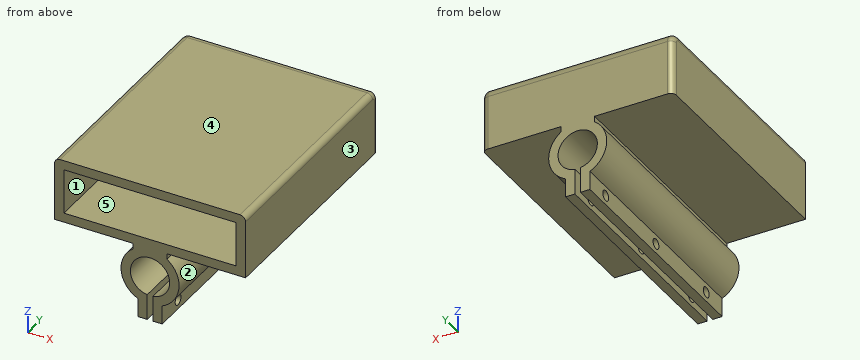
```python
from build123d import *

# Parameters (mm, degrees)
PAD_DEPTH       = 125
SKETCH001_W     = 92
SKETCH001_H     = 24
POCKET_DEPTH    = 120
FILLET_R        = 5
FILLET001_R     = 3
FILLET002_R     = 3
SKETCH002_R     = 2.75
POCKET001_DEPTH = 57.501


with BuildPart() as part:
    # Sketch → Pad (new body)
    with BuildSketch(Plane.XZ):
        with BuildLine():
            ThreePointArc((1.5, -26.011734), (0, -5.119429), (-1.5, -26.011734))
            Line((-1.5, -26.011734), (-1.5, -39.690677))
            Line((-1.5, -39.690677), (-6.5, -39.690677))
            Line((-6.5, -39.690677), (-6.5, -29.690677))
            ThreePointArc((-9, -3), (-15.432451, -17.06492), (-6.5, -29.690677))
            Line((-9, -3), (-9, 0))
            Line((-9, 0), (-51, 0))
            Line((-51, 0), (-51, 34))
            Line((-51, 34), (51, 34))
            Line((51, 0), (51, 34))
            Line((9, 0), (51, 0))
            Line((9, -3), (9, 0))
            ThreePointArc((6.5, -29.690677), (15.432451, -17.06492), (9, -3))
            Line((6.5, -39.690677), (6.5, -29.690677))
            Line((1.5, -39.690677), (6.5, -39.690677))
            Line((1.5, -26.011734), (1.5, -39.690677))
        make_face()
    extrude(amount=PAD_DEPTH)

    # Sketch001 (on Face18 of Pad) → Pocket (cut)
    with BuildSketch(Plane.XZ.offset(125)):
        with Locations((0, 17)):
            Rectangle(SKETCH001_W, SKETCH001_H)
    extrude(amount=-POCKET_DEPTH, mode=Mode.SUBTRACT)

    # Fillet
    fillet_edges = [part.edges().sort_by_distance(p)[0] for p in [
        (0, 0, 34),
    ]]
    fillet(fillet_edges, radius=FILLET_R)

    # Fillet001
    fillet001_edges = [part.edges().sort_by_distance(p)[0] for p in [
        (51, 0, 14.5),
    ]]
    fillet(fillet001_edges, radius=FILLET001_R)

    # Fillet002
    fillet002_edges = [part.edges().sort_by_distance(p)[0] for p in [
        (-51, 0, 14.5),
    ]]
    fillet(fillet002_edges, radius=FILLET002_R)

    # Sketch002 (on Face12 of Fillet002) → Pocket001 (cut, through all)
    with BuildSketch(Plane(origin=(6.5, 0, 0), x_dir=(0, 0, 1), z_dir=(1, 0, 0))):
        with Locations((-34.690677, 110)):
            Circle(SKETCH002_R)
        with Locations((-34.690677, 62.5)):
            Circle(SKETCH002_R)
        with Locations((-34.690677, 15)):
            Circle(SKETCH002_R)
    extrude(amount=-POCKET001_DEPTH, mode=Mode.SUBTRACT)


solid = part.part
```
Check sheet for the modelled part. Datum: model origin and axes. Units: mm. Face numbers are marked on the shaded views. A direction names the side the tool comes from. Round coordinates to 2 decimals unless told otherwise and drop trailing zeros. Order: outer loops, then holes, each group sorted by start corner. A loop starts at its lowest first (then second) coordinate and runs counter-clockwise, first axis right, second up.
1) Section check A-A (y = -110). Give the number of separate pieces and of enclosed holes in the cut face, and give its area (3 significant figures).
2) Tool access check on the marked faces 1 and 2. Record the directions out of +Z, -Z, +X, -X, +Y, -Y that give a thin tool (end or side, any length) a straight path to the whole face; none if there is none.
3) Mould release check, pull along X, two halves, no side actions. Record for the marked faces 3, 4 and 5: +X half, -X half, draft (parallel to the pull), parting line (faces both ways), or undercut.
4) Scan lines: line 1 (X direction, y = -88, z = 19); line 2 (Z direction, x = 30, y = -71); line 3 (X direction, y = -115.5, z = -35.5). Record each from-to range of solid material in increasing order.
5) Section check B-B (y = -25). Record the boundary of the cut face in (x, z), and give its area (3 significant figures).
6) Section check D-D (x = -29.5). Record the boundary of the cut face in (y, z).
7) Section check C-C (z = 13.5). Record the boundary of the cut face in (x, y).
8) Go/stop test with flat-tipped pins: pin 1 Ø11 at (y, z) = (-78, -36) entering from -X; pin 2 Ø8 at (y, z) = (-85.5, -12.5) entering from +X; pin 3 Ø5 at (x, y) = (12, -62.5) entering from -Z; pin 4 Ø5 at (y, z) = (-110, -34.69) entering from -X. Record where each tip stops, or that it passes through.
Result:
1. separate pieces: 3
1. enclosed holes: 1
1. area: 1,700 mm2
2. face 1: -Y
2. face 2: +X, +Y, -Y
3. face 3: +X half
3. face 4: draft
3. face 5: undercut
4. line 1: x = -51 to -46, 46 to 51
4. line 2: z = 0 to 5, 29 to 34
4. line 3: x = -6.5 to -1.5, 1.5 to 6.5
5. outline: (-51, 0) - (-9, 0) - (-9, -3) arc R15.5 ccw to (-6.5, -29.69) - (-6.5, -39.69) - (-1.5, -39.69) - (-1.5, -26.01) arc R10.5 cw (long way) to (1.5, -26.01) - (1.5, -39.69) - (6.5, -39.69) - (6.5, -29.69) arc R15.5 ccw to (9, -3) - (9, 0) - (51, 0) - (51, 31) arc R3 ccw to (48, 34) - (-48, 34) arc R3 ccw to (-51, 31) - close; hole (-46, 5) - (46, 5) - (46, 29) - (-46, 29) - close
5. area: 1,760 mm2
6. outline: (-125, 0) - (0, 0) - (0, 29) arc R5 ccw to (-5, 34) - (-125, 34) - (-125, 29) - (-5, 29) - (-5, 5) - (-125, 5) - close
7. outline: (-51, -125) - (-46, -125) - (-46, -5) - (46, -5) - (46, -125) - (51, -125) - (51, -3) arc R3 ccw to (48, 0) - (-48, 0) arc R3 ccw to (-51, -3) - close
8. pin 1: stops at x = -6.5
8. pin 2: stops at x = 15.5
8. pin 3: stops at z = -27.87
8. pin 4: passes through
